Input: dimensioned drawing with shaded views. Units: mm. Origin: part minimum x, y, z. Round coordinates to 2 decimals unless told otherwise and drop trailing zeros. Loops run counter-clockwise (first coordinate to the right, second up) from the corner with the lowest first, then second, coordinate; pieces in that order, holes last. Notation, with made-up numbers: (25.5, 54.5) - (36.5, 54.5) arc R23 cw to (36.5, 77.5) - close; hole circle Ø8 at (-37, 7). An arc over 180 degrees is marked (long way). Answer as a JSON object with one key per item and string values. Group by question number.
Item 1: First-contact query: pin 1 (3 mm diameter, centred on x = 3, y = 3, fed in from +Z); pin 2 (1 mm diameter, centred on y = 1.5, z = 2, fed in from +X). Flat tips, straight axial feed; report the tip coordinate or a pass-through.
Item 2: Line query: line 1 (Y direction, x = 23, z = 2.25); line 2 (X direction, y = 1.75, z = 2.25) (1 decimal); line 3 (X direction, y = 3.75, z = 0.95) (1 decimal). Output: solid intervals per line, ascending.
Item 3: Section D-D (y = 1.5). Return the cut outline in (x, z).
Item 4: Section C-C (y = 3.25). Return the cut outline in (x, z).
Item 5: Section B-B (x = 22.75). Return the cut outline in (y, z), plus the area to 3 significant figures.
Item 6: Section A-A (z = 0.85). Count the separate pieces of the cut face and the enclosed holes in it, plus the area to 3 significant figures.
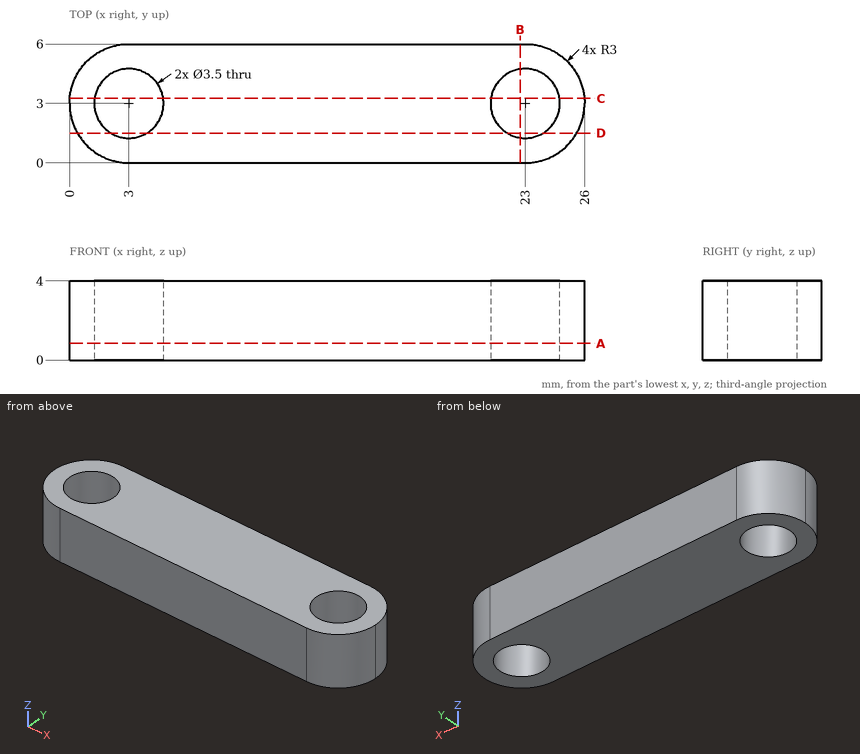
Values:
{
 "1": {"pin 1": "passes through", "pin 2": "stops at x = 25.83"},
 "2": {"line 1": "y = 0 to 1.25, 4.75 to 6", "line 2": "x = 0.3 to 1.8, 4.2 to 21.8, 24.2 to 25.7", "line 3": "x = 0.1 to 1.4, 4.6 to 21.4, 24.6 to 25.9"},
 "3": {"outline": "(0.4, 0) - (2.1, 0) - (2.1, 4) - (0.4, 4) - close; (3.9, 0) - (22.1, 0) - (22.1, 4) - (3.9, 4) - close; (23.9, 0) - (25.6, 0) - (25.6, 4) - (23.9, 4) - close"},
 "4": {"outline": "(0.01, 0) - (1.27, 0) - (1.27, 4) - (0.01, 4) - close; (4.73, 0) - (21.27, 0) - (21.27, 4) - (4.73, 4) - close; (24.73, 0) - (25.99, 0) - (25.99, 4) - (24.73, 4) - close"},
 "5": {"outline": "(0, 0) - (1.27, 0) - (1.27, 4) - (0, 4) - close; (4.73, 0) - (6, 0) - (6, 4) - (4.73, 4) - close", "area": "10.1 mm^2"},
 "6": {"separate pieces": "1", "enclosed holes": "2", "area": "129 mm^2"}
}
